Check sheet for the modelled part. Datum: model origin and axes. Units: mm. A direction names the side the tool comes from. Round coordinates to 2 decimals unless told otherwise and drop trailing zeros. Write each loop counter-clockwise with the first axis right and the second up, starting at its lowest first coordinate (ties: lowest second). Pieces come first, ordered by that corner, then holes. Notation, with made-up numbers: (18.25, 64.5) - (32.25, 64.5) arc R13 cw to (32.25, 82.5) - close; hole circle Ø6 at (-23, 52.25). An arc over 180 degrees is marked (long way). Answer as a JSON object with one key per item and string values. Group by question number.
Item 1: Thickness scan on line 1 (Y direction, x = 68, z = 3); line 2 (X direction, y = 56, z = 3); line 3 (Y direction, x = 77.5, z = 6.75). Record the ranges inside material, lowest first.
Item 2: Set-up check for faces 4 (the flat face through (72.14, 51.96, 16)), 5 (the flat face through (75.645, 47.197, 7.888)), 6 (the flat face through (38.6, 63.2, 1)): record each of +Z, -Z, +X, -X, +Y, -Y from which the full face is reachable in a straight line by a thin tool's end or side.
Item 3: Release check for a two-part mould opening along X. For faces 1 (the cylindrical face through (75.64, 76.155, 7.888)), 2 (the flat face through (74.185, 44.886, 7.888)), 3 (the cylindrical face through (60.207, 76.045, 7.888)) record: pulls with the +X half, pulls with the -X half, needs draft (parallel to the pull), parting line crosses it, or undercut.
Item 4: Sectioned sample at B-B on y = 50.5. Record the boundary of the cut face in (x, z), plus the area to 3 significant figures.
Item 5: Gauge pin test, flat ends, axial feed: P1, Ø0.6, axis at x = 36, z = 0.5, coming from the -Y side; P2, Ø1, axis at y = 58, z = 14, coming from the -X side; P3, Ø6, axis at y = 64.5, z = 11, coming from the +X side. Record the tip position at first contact, or that the pin passes through.
Item 6: Sectioned sample at A-A on x = 77. Record the boundary of the cut face in (y, z).
Item 7: Sectioned sample at C-C on z = 4. Count the separate pieces of the cut face and the enclosed holes in it, plus the area to 3 significant figures.
```python
from build123d import *

# Parameters (mm, degrees)
SKETCH1_R           = 0.9999999999999983
SKETCH1_R_2         = 0.9999999999999925
BOSS_EXTRUDE1_DEPTH = 16
SKETCH2_R           = 3.500000000000001
BOSS_EXTRUDE3_DEPTH = 1
FILLET1_R           = 1


with BuildPart() as part:
    # Sketch1 → Boss-Extrude1 (new body)
    with BuildSketch(Plane.XY):
        with BuildLine():
            ThreePointArc((55.89259723337368, 76.62547740283708), (55.73949455446561, 76.6384916731646), (55.58638884526515, 76.65147024516648))
            Line((55.586388845264466, 76.65147024517492), (40.05447850145701, 72.83576058817667))
            ThreePointArc((40.054478501457005, 72.83576058817668), (32.85162294085296, 64.37296720932677), (38.606783148321924, 54.86622586508078))
            Line((38.60678314832193, 54.86622586508078), (55.19963694216289, 47.81802020858516))
            ThreePointArc((55.19963694216289, 47.81802020858516), (57.2484781716781, 47.11230292338465), (59.37571808447544, 46.69921985208524))
            Line((59.375718084475444, 46.69921985208528), (71.42380227491209, 45.2239648632993))
            ThreePointArc((71.42380227491209, 45.22396486329929), (71.86683077979774, 45.14046516807511), (72.31691713492577, 45.1146053890486))
            Line((72.31691713492577, 45.11460538904862), (76.10592748748196, 44.65065142451647))
            Line((76.10592748748196, 44.65065142451647), (84.55064590566833, 43.80531307650732))
            ThreePointArc((84.55064590566833, 43.805313076507325), (101.48886829968637, 57.421563726672275), (88.16345849536586, 74.58953137529774))
            ThreePointArc((88.16345849536584, 74.58953137529784), (75.46175434404655, 76.17510896963688), (62.73170883439283, 77.5142452500271))
            ThreePointArc((62.73170883439284, 77.5142452500271), (59.262094380223, 77.45506508921636), (55.89259723337367, 76.62547740283709))
        make_face()
        with BuildLine():
            ThreePointArc((59.557725585447635, 48.18813669728694), (57.63650253765193, 48.561246371899415), (55.78608310126676, 49.19862909689187))
            Line((55.78608310126676, 49.19862909689187), (39.19322930742587, 56.24683475338757))
            ThreePointArc((39.19322930742587, 56.246834753387574), (34.34677860639931, 64.25251167485804), (40.41234118375017, 71.37907452020546))
            Line((40.41234118375017, 71.37907452020545), (57.91952888483379, 75.68004868881708))
            ThreePointArc((57.91952888483379, 75.6800486888171), (60.24003267144862, 76.04713848925702), (62.589247617854994, 76.02102564066264))
            ThreePointArc((62.589247617854994, 76.02102564066263), (67.20240478832663, 75.56451764159874), (71.81223656797964, 75.07557020476702))
            Line((71.81223656797964, 75.07557020476696), (71.64178678398153, 73.59342993840335))
            ThreePointArc((71.64178678398147, 73.59342993840333), (71.65659417306406, 73.58005511327626), (71.67138433211107, 73.56666123728807))
            ThreePointArc((71.67138433211102, 73.56666123728805), (74.42615226207305, 69.25624682134095), (78.53896424094067, 72.29815352793712))
            Line((78.53896424094067, 72.29815352793712), (78.76640123459923, 74.2758241266035))
            ThreePointArc((78.76640123459923, 74.27582412660365), (83.36688258884593, 73.70556283958138), (87.96323868046352, 73.10295408981267))
            ThreePointArc((87.96323868046352, 73.10295408981273), (99.9990926972691, 57.59640266524784), (84.70005311557539, 45.2978536909054))
            Line((84.70005311557539, 45.29785369090539), (76.25533469738902, 46.14319203891454))
            ThreePointArc((76.25533469738902, 46.14319203891455), (75.56489776696996, 46.20456627537837), (74.87326752192872, 46.25058318457722))
            ThreePointArc((74.87326752192874, 46.25058318457718), (74.89840357996093, 46.278324250051526), (74.92324149301305, 46.306332573854725))
            Line((74.92324149301308, 46.30633257385466), (75.52663710324227, 46.23243513010978))
            Line((75.52663710324227, 46.2324351301098), (75.76626292593124, 48.189054495825076))
            ThreePointArc((75.76626292593126, 48.189054495825076), (72.46724927571279, 52.11013899674976), (68.79305098926964, 48.53821211065343))
            ThreePointArc((68.79305098926967, 48.53821211065338), (68.77357245948804, 48.527397725244626), (68.75407840556292, 48.51661134884714))
            Line((68.75407840556268, 48.51661134884727), (68.57854942467414, 47.08336263050453))
            Line((68.57854942467414, 47.08336263050455), (59.55772558544767, 48.18813669728721))
        make_face(mode=Mode.SUBTRACT)
        with Locations((75.06188190763086, 72.69802656701884)):
            Circle(SKETCH1_R, mode=Mode.SUBTRACT)
        with Locations(Location((72.29221908664718, 48.614518246022456, 0), (0, 0, 180))):
            Circle(SKETCH1_R_2, mode=Mode.SUBTRACT)
    extrude(amount=BOSS_EXTRUDE1_DEPTH)

    # Sketch2 → Boss-Extrude3 (add)
    with BuildSketch(Plane(origin=(0, 0, 0), x_dir=(-1, 0, 0), z_dir=(0, 0, -1))):
        with BuildLine():
            Line((-34.38368822278696, 64.61008215769137), (-36.91261524278492, 64.61008215769137))
            ThreePointArc((-36.91261524278492, 64.61008215769137), (-38.431854859454894, 67.49916945421737), (-41.3209421559809, 69.01840907088734))
            Line((-41.3209421559809, 69.01840907088734), (-41.3209421559809, 71.60228965777424))
            Line((-41.3209421559809, 71.60228965777424), (-43.3209421559809, 72.09362775753603))
            Line((-43.3209421559809, 72.09362775753601), (-43.3209421559809, 69.01840907088734))
            ThreePointArc((-43.3209421559809, 69.01840907088734), (-47.8209421559809, 63.61008215769136), (-43.3209421559809, 58.201755244495374))
            Line((-43.3209421559809, 58.20175524449537), (-43.3209421559809, 54.49349145216626))
            Line((-43.320942155980916, 54.493491452166296), (-41.3209421559809, 55.343038581800116))
            Line((-41.3209421559809, 55.343038581800116), (-41.3209421559809, 58.20175524449537))
            ThreePointArc((-41.3209421559809, 58.201755244495374), (-38.431854859454894, 59.72099486116535), (-36.91261524278492, 62.61008215769136))
            Line((-36.91261524278492, 62.61008215769136), (-34.38368822278692, 62.61008215769136))
            ThreePointArc((-34.383688222786944, 62.6100821576915), (-34.32094215598073, 63.61008215769144), (-34.38368822278696, 64.61008215769137))
        make_face()
        with Locations((-42.3209421559809, 63.61008215769136)):
            Circle(SKETCH2_R, mode=Mode.SUBTRACT)
    extrude(amount=-BOSS_EXTRUDE3_DEPTH)

    # Fillet1
    # the kernel refuses this fillet: 1 mm, written as the material it adds along each edge
    with BuildSketch(Plane(origin=(43.3209421559809, 69.01840907088734, 0), x_dir=(0, 1, 0), z_dir=(0, 0, 1))) as fillet1_piece_1:
        with BuildLine():
            CenterArc((0.7763315252305034, -1), FILLET1_R, 90, 72.07978686060775)
            ThreePointArc((-0.17515438837357067, -0.6923076923076934), (-0.07632915836303766, -0.3489996080267872), (0, 0))
            Line((0, 0), (0.7763315252305034, 0))
        make_face()
    extrude(amount=1)
    with BuildSketch(Plane(origin=(43.3209421559809, 72.09362775753601, 0), x_dir=(0.9711240453142455, 0.23857512152882837, 0), z_dir=(0, 0, 1))) as fillet1_piece_2:
        with BuildLine():
            CenterArc((FILLET1_R * 0.784065518865, -FILLET1_R), FILLET1_R, 90.00000000000067, 76.19754186301965)
            Line((-FILLET1_R * 0.18705852645, -FILLET1_R * 0.761424878471), (0, 0))
            Line((0, 0), (FILLET1_R * 0.784065518865, 0))
        make_face()
    extrude(amount=1)
    with BuildSketch(Plane(origin=(41.3209421559809, 71.60228965777424, 0), x_dir=(-0.9693820258646232, -0.24555750432556298, 0), z_dir=(0, 0, 1))) as fillet1_piece_3:
        with BuildLine():
            CenterArc((1.2846787374655042, 0.9991324752357655), FILLET1_R, 165.78521711475895, 106.60154959902064)
            Line((0.31529671160088446, 1.2446899795613422), (0.21835850901442075, 1.2692457299938988))
            Line((0.21835850901442075, 1.2692457299938988), (-0.0969382025864637, 0.02455575043255665))
            Line((-0.0969382025864637, 0.02455575043255665), (-0.00071963623293713, -0.09999741058494188))
            ThreePointArc((-0.00071963623293713, -0.09999741058494188), (0.9348739670397286, -0.10673045549363312), (1.3304881173388574, -0.09991324752357857))
            Line((1.3304881173388574, -0.09991324752357857), (1.3263236282594648, 2e-17))
        make_face()
    extrude(amount=1)
    with BuildSketch(Plane(origin=(34.38368822278696, 64.61008215769137, 0), x_dir=(0.20605308678190415, 0.9785408143903089, 0), z_dir=(0, 0, 1))) as fillet1_piece_4:
        with BuildLine():
            CenterArc((1.2317903608426914, -0.9966225018240038), FILLET1_R, 85.28960309121933, 106.60154959901973)
            Line((0.25324954645238257, -1.202675588605908), (0, 0))
            ThreePointArc((0, 0), (0.6569548591160989, 0.02701998540798078), (1.3139097182321993, 1e-17))
        make_face()
    extrude(amount=1)
    with BuildSketch(Plane(origin=(34.38368822278693, 62.61008215769143, 0), x_dir=(0.206053086781914, -0.9785408143903069, 0), z_dir=(0, 0, 1))) as fillet1_piece_5:
        with BuildLine():
            CenterArc((1.231790360842777, 0.9966225018240046), FILLET1_R, 168.10884730976036, 106.60154959901973)
            Line((0.2532495464524701, 1.2026755886059186), (0, 0))
            ThreePointArc((0, 0), (0.6569548591161378, -0.02701998540797386), (1.3139097182322748, -1e-17))
        make_face()
    extrude(amount=1)
    with BuildSketch(Plane(origin=(41.3209421559809, 58.201755244495374, 0), x_dir=(0, -1, 0), z_dir=(0, 0, 1))) as fillet1_piece_6:
        with BuildLine():
            CenterArc((0.7763315252304963, -1), FILLET1_R, 90, 72.07978686060738)
            ThreePointArc((-0.17515438837357777, -0.6923076923076863), (-0.07632915836303766, -0.3489996080267801), (0, 0))
            Line((0, 0), (0.7763315252304963, 0))
        make_face()
    extrude(amount=1)
    with BuildSketch(Plane(origin=(41.3209421559809, 55.343038581800116, 0), x_dir=(-0.9204059255379603, 0.390964106069356, 0), z_dir=(0, 0, 1))) as fillet1_piece_7:
        with BuildLine():
            CenterArc((FILLET1_R * 1.51125070741, -FILLET1_R), FILLET1_R, 89.99999999999925, 113.0145022041728)
            Line((FILLET1_R * 0.590844781867, -FILLET1_R * 1.39096410607), (0, 0))
            Line((0, 0), (FILLET1_R * 1.51125070741, 3e-17))
        make_face()
    extrude(amount=1)
    with BuildSketch(Plane(origin=(43.32094215598091, 54.49349145216628, 0), x_dir=(0.9204059255379384, -0.3909641060694075, 0), z_dir=(0, 0, 1))) as fillet1_piece_8:
        with BuildLine():
            CenterArc((FILLET1_R * 0.661703577772, FILLET1_R), FILLET1_R, 203.01450220417283, 66.98549779582959)
            Line((-FILLET1_R * 0.258702347766, FILLET1_R * 0.609035893931), (0, 0))
            Line((0, 0), (FILLET1_R * 0.661703577772, 0))
        make_face()
    extrude(amount=1)
    with BuildSketch(Plane(origin=(36.91261524278492, 64.61008215769137, 0), x_dir=(-1, 0, 0), z_dir=(0, 0, 1))) as fillet1_piece_9:
        with BuildLine():
            CenterArc((0.7763315252305034, -1), FILLET1_R, 90, 72.07978686060696)
            ThreePointArc((-0.17515438837357067, -0.6923076923076792), (-0.07632915836303766, -0.348999608026773), (0, 0))
            Line((0, 0), (0.7763315252305034, 0))
        make_face()
    extrude(amount=1)
    with BuildSketch(Plane(origin=(43.3209421559809, 58.201755244495374, 0), x_dir=(0, -1, 0), z_dir=(0, 0, 1))) as fillet1_piece_10:
        with BuildLine():
            CenterArc((0.7763315252305034, 1), FILLET1_R, 197.92021313939225, 72.07978686060778)
            ThreePointArc((-0.17515438837357067, 0.6923076923076934), (-0.07632915836303766, 0.3489996080267872), (0, 0))
            Line((0, 0), (0.7763315252305034, 0))
        make_face()
    extrude(amount=1)
    with BuildSketch(Plane(origin=(41.3209421559809, 69.01840907088734, 0), x_dir=(-0.9694541372423533, -0.24527265600487255, 0), z_dir=(0, 0, 1))) as fillet1_piece_11:
        with BuildLine():
            CenterArc((0.779041242108754, -0.9978904650112504), FILLET1_R, 93.72226572150103, 72.07978686060773)
            Line((-0.1904128951335993, -0.7526178090063779), (0, 0))
            ThreePointArc((0, 0), (0.35706056929984037, -0.01160244243811416), (0.7141211385996942, -1e-17))
        make_face()
    extrude(amount=1)
    with BuildSketch(Plane(origin=(36.91261524278492, 62.61008215769136, 0), x_dir=(0.2452726560048725, -0.9694541372423532, 0), z_dir=(0, 0, 1))) as fillet1_piece_12:
        with BuildLine():
            CenterArc((0.7790412421087539, -0.9978904650112503), FILLET1_R, 93.72226572150103, 72.07978686060773)
            Line((-0.19041289513359927, -0.7526178090063779), (0, 0))
            ThreePointArc((0, 0), (0.3570605692998403, -0.01160244243811414), (0.7141211385996941, 2e-17))
        make_face()
    extrude(amount=1)


solid = part.part
```
Completed:
{
 "1": {"line 1": "45.64 to 47.15, 75.48 to 76.99", "line 2": "36.63 to 39.77, 99.72 to 101.25", "line 3": "44.51 to 46.02, 70.19 to 75.94"},
 "2": {"face 4": "+Z, +X, -X, +Y, -Y", "face 5": "+Z, -Z", "face 6": "+Z"},
 "3": {"face 1": "pulls with the +X half", "face 2": "pulls with the -X half", "face 3": "undercut"},
 "4": {"outline": "(48.89, 0) - (52.72, 0) - (52.72, 16) - (48.89, 16) - close; (69.34, 0) - (75.24, 0) - (75.24, 16) - (69.34, 16) - close; (97.04, 0) - (98.9, 0) - (98.9, 16) - (97.04, 16) - close", "area": "186 mm²"},
 "5": {"P1": "y = 56.26", "P2": "x = 34.31", "P3": "x = 101.43"},
 "6": {"outline": "(44.56, 0) - (46.07, 0) - (46.07, 16) - (44.56, 16) - close; (69.78, 0) - (76, 0) - (76, 16) - (69.78, 16) - close"},
 "7": {"separate pieces": "1", "enclosed holes": "3", "area": "305 mm²"}
}
